Part model, mm, in its own coordinate system. Face numbers are marked on the shaded views. A direction names the side the tool comes from. Round coordinates to 2 decimals unless told otherwise and drop trailing zeros. Write each loop counter-clockwise with the first axis right and the second up, starting at its lowest first coordinate (ties: lowest second). Pieces come first, ordered by that corner, then holes.
1) Saw through at C-C on x = 21.5. Write the cut outline in (y, z), and give its area (3 significant figures).
2) Which spindle directions (+Z, -Z, +X, -X, +Y, -Y) get a long thin tool onto all of the face, cutting with end or side? Do the marked faces 1 and 2. Say none if no direction does.
3) Drill centre lines: L1, parallel to Z at x = -4.5, y = 10.5; L2, parallel to Z at x = 24, y = 21; L3, parallel to Y at x = 7.5, z = 53. Where is each one in solid material? Low to high.
4) Flat gauge pins, fed straight in: pin 1 (4 mm diameter, centred on x = 1.5, z = 17.5, fed in from +Y); pin 2 (1.5 mm diameter, centred on y = 16, z = 13, fed in from +X); pin 3 (7.5 mm diameter, centred on x = 29.73, y = 16.95, fed in from +Z). Where does each tip first touch, or does it go through?
5) Saw through at B-B on z = 45.5. Write the cut outline in (x, y), and give its area (3 significant figures).
6) Saw through at D-D on z = 35. Write the cut outline in (x, y), and give its area (3 significant figures).
7) Saw through at A-A on x = 0. Write the cut outline in (y, z).
```python
from build123d import *

# Parameters (mm, degrees)
F1_DEPTH = 12.7
F2_R     = 3.175
F3_DEPTH = 25.4
F4_W     = 15.6316435844
F4_H     = 44.45
F6_SIZE  = 2.54
F9_R     = 2.54


# Not quite as in the source:
# - a feature names something its author has since deleted; it is built from what else it names


with BuildPart() as f1:
    # F0 (on Top) → F1 (new body)
    with BuildSketch(Plane.XY):
        Polygon((27.94, 25.4), (-27.94, 25.4), (-38.1, 25.4), (-38.1, 15.24), (-38.1, -15.24), (-38.1, -25.4), (-27.94, -25.4), (27.94, -25.4), (38.1, -25.4), (38.1, -15.24), (38.1, 15.24), (38.1, 25.4), align=None)
    extrude(amount=F1_DEPTH)

    # F2 (on face) → F3 (cut)
    with BuildSketch(Plane.XY.offset(12.7)):
        with Locations((-30.4814037019, 18.666748425)):
            Circle(F2_R)
        with Locations((29.7281444444, 16.9542004048)):
            Circle(F2_R)
        with Locations((30.147915706, -18.4229128063)):
            Circle(F2_R)
        with Locations((-30.2868466824, -18.3251220733)):
            Circle(F2_R)
    extrude(amount=-F3_DEPTH, mode=Mode.SUBTRACT)

    # F4 (on Front) → F5 (revolve)
    with BuildSketch(Plane.XZ):
        with Locations((7.8158217922, 34.925)):
            Rectangle(F4_W, F4_H)
    revolve(axis=Axis((0, 0, 34.925), (0, 0, -1)))

    # F6
    f6_edges = [f1.edges().sort_by_distance(p)[0] for p in [
        (0, -25.4, 12.7),
        (38.1, 0, 12.7),
        (0, 25.4, 12.7),
        (-38.1, 0, 12.7),
    ]]
    chamfer(f6_edges, length=F6_SIZE)

    # F7 (on Front) → F8 (revolve, cut)
    with BuildSketch(Plane.XZ):
        with BuildLine():
            Line((19.2013573515, 37.423838021), (9.0413573515, 37.423838021))
            Line((9.0413573515, 37.423838021), (9.0413573515, 32.343838021))
            ThreePointArc((9.0413573515, 32.343838021), (9.7853061273, 30.5477867968), (11.5813573515, 29.803838021))
            Line((11.5813573515, 29.803838021), (19.2013573515, 29.803838021))
            Line((19.2013573515, 29.803838021), (19.2013573515, 37.423838021))
        make_face()
    revolve(axis=Axis((0, 0, 12.7), (0, 0, 1)), mode=Mode.SUBTRACT)

    # F9
    f9_edges = [f1.edges().sort_by_distance(p)[0] for p in [
        (-15.631644, 0, 12.7),
        (-15.631644, 0, 57.15),
        (15.631644, 0, 21.251919),
        (-15.631644, 0, 29.803838),
        (-15.631644, 0, 37.423838),
        (15.631644, 0, 47.286919),
    ]]
    fillet(f9_edges, radius=F9_R)


solid = f1.part
```
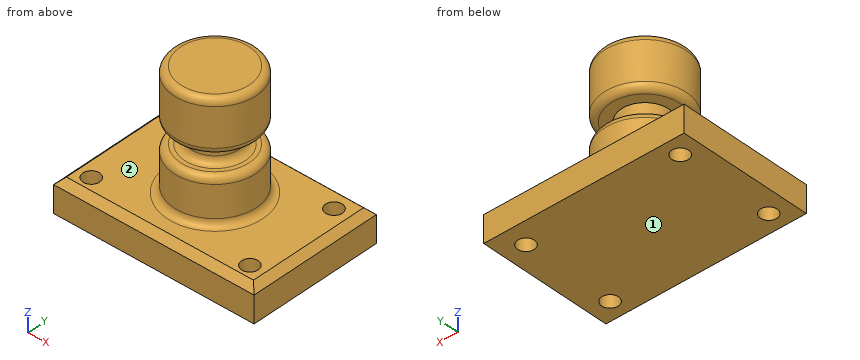
Completed:
1. outline: (-25.4, 0) - (25.4, 0) - (25.4, 10.16) - (22.86, 12.7) - (-22.86, 12.7) - (-25.4, 10.16) - close
1. area: 639 mm2
2. face 1: -Z, +X, -X, +Y, -Y
2. face 2: +Z
3. L1: z = 0 to 29.81, 37.42 to 57.15
3. L2: z = 0 to 12.7
3. L3: y = -13.71 to 13.71
4. pin 1: stops at y = 15.63
4. pin 2: stops at x = 36.01
4. pin 3: stops at z = 12.7
5. outline: circle Ø31.26 at (0, 0)
5. area: 768 mm2
6. outline: circle Ø18.08 at (0, 0)
6. area: 257 mm2
7. outline: (-25.4, 0) - (25.4, 0) - (25.4, 10.16) - (22.86, 12.7) - (18.17, 12.7) arc R2.54 cw to (15.63, 15.24) - (15.63, 27.26) arc R2.54 ccw to (13.09, 29.8) - (11.58, 29.8) arc R2.54 cw to (9.04, 32.34) - (9.04, 37.42) - (13.09, 37.42) arc R2.54 ccw to (15.63, 39.96) - (15.63, 54.61) arc R2.54 ccw to (13.09, 57.15) - (-13.09, 57.15) arc R2.54 ccw to (-15.63, 54.61) - (-15.63, 39.96) arc R2.54 ccw to (-13.09, 37.42) - (-9.04, 37.42) - (-9.04, 32.34) arc R2.54 cw to (-11.58, 29.8) - (-13.09, 29.8) arc R2.54 ccw to (-15.63, 27.26) - (-15.63, 15.24) arc R2.54 cw to (-18.17, 12.7) - (-22.86, 12.7) - (-25.4, 10.16) - close
